Geometry: final body of the model. Coordinates: model frame, mm. Give positions to 0.01 mm unless a question says otherwise; leave off trailing zeros. Write each loop counter-clockwise with the first axis right and the second up, starting at its lowest first coordinate (ties: lowest second). Pieces come first, ordered by that corner, then holes. Notation, with made-up numbers: M -28,-13.75 L 6,-13.75 A12 ccw 6,-8.75 Z; hole C 46.25,-19 d5. An arc over 180 degrees is marked long. One line per question, with ' | ' between items.
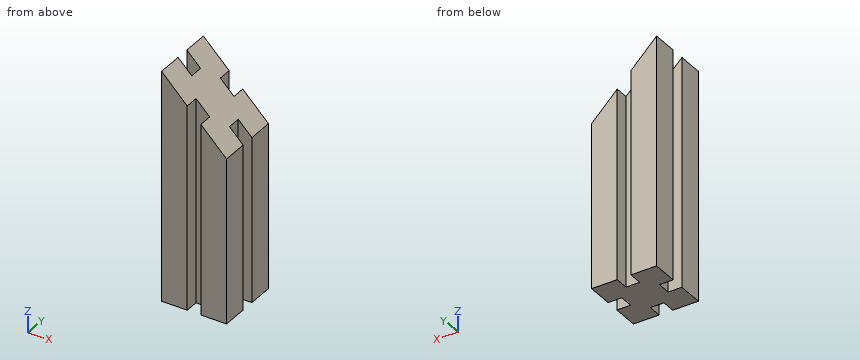
from build123d import *

# Parameters (mm, degrees)
PROFILE_DEPTH     = 135
MITER1_DEPTH      = 138.66192284
MITER1_DEPTH_BACK = 138.66192284


with BuildPart() as part:
    # Sketch1 → Profile (new body)
    with BuildSketch(Plane.XY):
        Polygon((-19.05, -19.05), (-4, -19.05), (-4, -11.05), (4, -11.05), (4, -19.05), (19.05, -19.05), (19.05, -4), (11.05, -4), (11.05, 4), (19.05, 4), (19.05, 19.05), (4, 19.05), (4, 11.05), (-4, 11.05), (-4, 19.05), (-19.05, 19.05), (-19.05, 4), (-11.05, 4), (-11.05, -4), (-19.05, -4), align=None)
    extrude(amount=PROFILE_DEPTH)

    # Sketch2 → Miter1 (cut, two sides: drawn at the far end of the back side and taken through both)
    with BuildSketch(Plane(origin=(0, 0, 0), x_dir=(1, 0, 0), z_dir=(0, 1, 0)).offset(-MITER1_DEPTH_BACK)):
        Polygon((-19.05, -135), (25, -90.95), (25, -145), align=None)
    extrude(amount=MITER1_DEPTH + MITER1_DEPTH_BACK, mode=Mode.SUBTRACT)


solid = part.part
(1) Material intervals for L1, parallel to X at y = 15.5, z = 24; L2, parallel to X at y = 0, z = 92.5, sorted ascending. Write a range as [from, to].
Working result:
L1: x = [-19.05, -4], [4, 19.05] | L2: x = [-11.05, 11.05]
(2) Cut plane C-C, the plane z = 109.5. Return loops of the section in (x, y).
Working result:
outline: M -19.05,-19.05 L -4,-19.05 L -4,-11.05 L 4,-11.05 L 4,-19.05 L 6.45,-19.05 L 6.45,19.05 L 4,19.05 L 4,11.05 L -4,11.05 L -4,19.05 L -19.05,19.05 L -19.05,4 L -11.05,4 L -11.05,-4 L -19.05,-4 Z
(3) First-contact query: P1, Ø8, axis at x = -6, y = -6, coming from the +Z side; P2, Ø10, axis at y = 8, z = 111, coming from the +X side; P3, Ø2.5, axis at y = -1, z = 82, coming from the -X side. Flat tips, straight axial feed; report the tip coordinate or a pass-through.
Working result:
P1: stops at z = 125.95 | P2: stops at x = 9.95 | P3: stops at x = -11.05
(4) Cut plane D-D, the plane x = -2.5. Return loops of the section in (y, z), then the cut area to 3 significant figures.
Working result:
outline: M -11.05,0 L 11.05,0 L 11.05,118.45 L -11.05,118.45 Z | area: 2,620 mm^2
(5) Cut plane A-A, the plane x = 14.5. Return loops of the section in (y, z), then the cut area to 3 significant figures.
Working result:
outline: M -19.05,0 L -4,0 L -4,101.45 L -19.05,101.45 Z; M 4,0 L 19.05,0 L 19.05,101.45 L 4,101.45 Z | area: 3,050 mm^2
(6) Cut plane B-B, the plane y = 13. Return loops of the section in (x, z).
Working result:
outline: M -19.05,0 L -4,0 L -4,119.95 L -19.05,135 Z; M 4,0 L 19.05,0 L 19.05,96.9 L 4,111.95 Z
